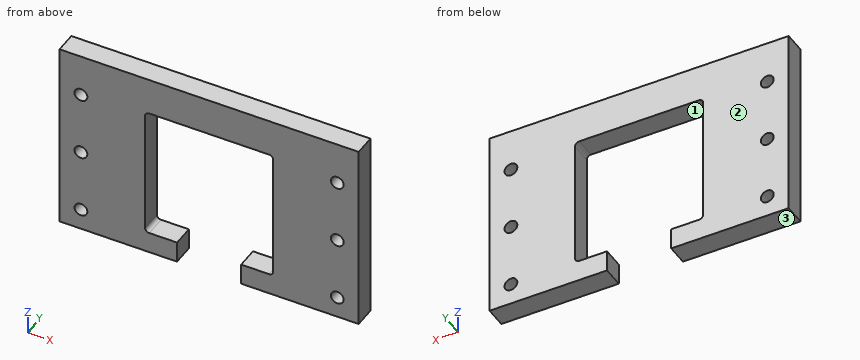
from build123d import *

# Parameters (mm, degrees)
SKETCH1_R           = 3.81
BOSS_EXTRUDE1_DEPTH = 12.7


with BuildPart() as part:
    # Sketch1 → Boss-Extrude1 (new body)
    with BuildSketch(Plane(origin=(0, 0, 0), x_dir=(1, 0, 0), z_dir=(0, 1, 0))):
        with BuildLine():
            Line((92.067570855, 107.193983746), (161.917570855, 107.193983746))
            Line((161.917570855, 107.193983746), (161.917570855, -7.106016254))
            Line((161.917570855, -7.106016254), (-15.882429145, -7.106016254))
            Line((-15.882429145, -7.106016254), (-15.882429145, 107.193983746))
            Line((-15.882429145, 107.193983746), (53.967570855, 107.193983746))
            Line((53.967570855, 107.193983746), (53.967570855, 94.493983746))
            Line((53.967570855, 94.493983746), (37.457570855, 94.493983746))
            ThreePointArc((37.457570855, 94.493983746), (35.661519631, 93.75003497), (34.917570855, 91.953983746))
            Line((34.917570855, 91.953983746), (34.917570855, 17.658983746))
            ThreePointArc((34.917570855, 17.658983746), (35.661519631, 15.862932521), (37.457570855, 15.118983746))
            Line((37.457570855, 15.118983746), (108.577570855, 15.118983746))
            ThreePointArc((108.577570855, 15.118983746), (110.373622079, 15.862932521), (111.117570855, 17.658983746))
            Line((111.117570855, 17.658983746), (111.117570855, 91.953983746))
            ThreePointArc((111.117570855, 91.953983746), (110.373622079, 93.75003497), (108.577570855, 94.493983746))
            Line((108.577570855, 94.493983746), (92.067570855, 94.493983746))
            Line((92.067570855, 94.493983746), (92.067570855, 107.193983746))
        make_face()
        with Locations(Location((-3.182429145, 94.493983746, 0), (0, 0, 270))):
            Circle(SKETCH1_R, mode=Mode.SUBTRACT)
        with Locations(Location((-3.182429145, 56.393983746, 0), (0, 0, 270))):
            Circle(SKETCH1_R, mode=Mode.SUBTRACT)
        with Locations(Location((-3.182429145, 18.293983746, 0), (0, 0, 270))):
            Circle(SKETCH1_R, mode=Mode.SUBTRACT)
        with Locations(Location((149.217570855, 94.493983746, 0), (0, 0, 90))):
            Circle(SKETCH1_R, mode=Mode.SUBTRACT)
        with Locations(Location((149.217570855, 56.393983746, 0), (0, 0, 90))):
            Circle(SKETCH1_R, mode=Mode.SUBTRACT)
        with Locations(Location((149.217570855, 18.293983746, 0), (0, 0, 90))):
            Circle(SKETCH1_R, mode=Mode.SUBTRACT)
    extrude(amount=BOSS_EXTRUDE1_DEPTH)


solid = part.part
CAD build for the part. Positions are in the model's coordinates, mm. Face numbers are marked on the shaded views. Round coordinates to 2 decimals unless told otherwise and drop trailing zeros. Write each loop counter-clockwise with the first axis right and the second up, starting at its lowest first coordinate (ties: lowest second). Pieces come first, ordered by that corner, then holes. Notation, with made-up numbers: M -12.5,55 L -6.5,55 A8 ccw -6.5,59 Z; hole C 76.25,9.5 d7. An arc over 180 degrees is marked long. Put each result on its own line as item: value. Start each with the question number.
1) Saw through at D-D, the plane y = 9.75. Write the cut outline in (x, z), and give its area (3 significant figures).
2) Saw through at B-B, the plane z = -65. Write the cut outline in (x, y).
3) Pull direction Z, two halves, no side cores. Call the marked faces 1, 2 and 3: pulls with the +Z half, pulls with the -Z half, needs draft (parallel to the pull), parting line crosses it, or undercut.
4) Saw through at A-A, the plane x = 101.5. Write the cut outline in (y, z), and give its area (3 significant figures).
5) Saw through at C-C, the plane x = 147.5. Write the cut outline in (y, z).
6) Drill centre lines: probe 1 along X at (y, z) = (2.5, -42); probe 2 along Z at (x, y) = (41.5, 9.25); probe 3 along X at (y, z) = (7.25, -18). Where is each one in solid material? Low to high. Write a range as [from, to].
7) Pin check, flat tips, straight feed: pin 1 Ø4 at (x, y) = (88, 9) entering from -Z; pin 2 Ø6 at (x, z) = (149.22, -18.29) entering from -Y. Stop position of each tip, or through.
Resolved:
1. outline: M -15.88,-107.19 L 53.97,-107.19 L 53.97,-94.49 L 37.46,-94.49 A2.54 cw 34.92,-91.95 L 34.92,-17.66 A2.54 cw 37.46,-15.12 L 108.58,-15.12 A2.54 cw 111.12,-17.66 L 111.12,-91.95 A2.54 cw 108.58,-94.49 L 92.07,-94.49 L 92.07,-107.19 L 161.92,-107.19 L 161.92,7.11 L -15.88,7.11 Z; hole C -3.18,-94.49 d7.62; hole C -3.18,-56.39 d7.62; hole C -3.18,-18.29 d7.62; hole C 149.22,-94.49 d7.62; hole C 149.22,-56.39 d7.62; hole C 149.22,-18.29 d7.62
1. area: 13,500 mm²
2. outline: M -15.88,0 L 34.92,0 L 34.92,12.7 L -15.88,12.7 Z; M 111.12,0 L 161.92,0 L 161.92,12.7 L 111.12,12.7 Z
3. face 1: undercut
3. face 2: needs draft
3. face 3: pulls with the -Z half
4. outline: M 0,-107.19 L 12.7,-107.19 L 12.7,-94.49 L 0,-94.49 Z; M 0,-15.12 L 12.7,-15.12 L 12.7,7.11 L 0,7.11 Z
4. area: 444 mm²
5. outline: M 0,-107.19 L 12.7,-107.19 L 12.7,-97.89 L 0,-97.89 Z; M 0,-91.09 L 12.7,-91.09 L 12.7,-59.79 L 0,-59.79 Z; M 0,-52.99 L 12.7,-52.99 L 12.7,-21.69 L 0,-21.69 Z; M 0,-14.89 L 12.7,-14.89 L 12.7,7.11 L 0,7.11 Z
6. probe 1: [-15.88, 34.92], [111.12, 161.92]
6. probe 2: [-107.19, -94.49], [-15.12, 7.11]
6. probe 3: [-15.88, -6.98], [0.62, 34.92], [111.12, 145.42], [153.02, 161.92]
7. pin 1: z = -15.12
7. pin 2: through
